```python
from build123d import *

# Parameters (mm, degrees)
CROQUIS1_R                 = 1.6
SALIENTE_EXTRUIR1_DEPTH    = 10
CORTAR_EXTRUIR1_DEPTH      = 8.1
CORTAR_EXTRUIR1_DEPTH_BACK = 8.1
CORTAR_EXTRUIR2_START      = 8.1
CROQUIS3_OUTSIDE_W         = 34.658
CROQUIS3_OUTSIDE_H         = 30.658
CROQUIS3_OUTSIDE_W_2       = 10
CROQUIS3_OUTSIDE_H_2       = 25.797501395
CORTAR_EXTRUIR2_DEPTH      = 8
CROQUIS4_W                 = 10
CROQUIS4_H                 = 8
SALIENTE_EXTRUIR3_DEPTH    = 3
CORTAR_EXTRUIR3_DEPTH      = 25.088378941
CORTAR_EXTRUIR3_DEPTH_BACK = 25.088378941
CROQUIS5_W                 = 8.1
CROQUIS5_H                 = 3.5
CROQUIS6_R                 = 4.5
CROQUIS6_R_2               = 1.6
SALIENTE_EXTRUIR4_DEPTH    = 3
CHAFL_N1_SIZE              = 1
CROQUIS7_R                 = 3.5
CORTAR_EXTRUIR4_DEPTH      = 3
SALIENTE_EXTRUIR8_START    = -1.9
CROQUIS8_R                 = 0.75
CROQUIS8_R_2               = 1.945
CROQUIS8_W                 = 23.65
CROQUIS8_H                 = 12.1
SALIENTE_EXTRUIR8_DEPTH    = 1.9
SALIENTE_EXTRUIR9_START    = 5
CROQUIS9_R                 = 1.945
SALIENTE_EXTRUIR9_DEPTH    = 5
CROQUIS10_W                = 23.280139212
CROQUIS10_H                = 3
SALIENTE_EXTRUIR10_DEPTH   = 11.4
CROQUIS11_R                = 1.945
SALIENTE_EXTRUIR11_DEPTH   = 2
REDONDEO1_R                = 3
CROQUIS12_W                = 4.35
CROQUIS12_H                = 6
CROQUIS12_R                = 0.75
SALIENTE_EXTRUIR12_DEPTH   = 2
CHAFL_N3_SIZE              = 2
CHAFL_N2_SIZE              = 1


# Some blends are built 0.0001 mm under size
with BuildPart() as part:
    # Croquis1 → Saliente-Extruir1 (new, symmetric)
    with BuildSketch(Plane.XY):
        with BuildLine():
            Line((-12.5, -15), (-5.566639674, 2.238866395))
            ThreePointArc((-5.566639674, 2.238866395), (0, 6), (5.566639674, 2.238866395))
            Line((5.566639674, 2.238866395), (12.5, -15))
            Line((12.5, -15), (-12.5, -15))
        make_face()
        Circle(CROQUIS1_R, mode=Mode.SUBTRACT)
    extrude(amount=SALIENTE_EXTRUIR1_DEPTH, both=True)

    # Croquis2 → Cortar-Extruir1 (cut, two sides: drawn at the far end of the back side and taken through both)
    with BuildSketch(Plane.XY.offset(-CORTAR_EXTRUIR1_DEPTH_BACK)):
        with BuildLine():
            Line((-12.5, -15), (-7.5, 0))
            ThreePointArc((-7.5, 0), (0, 7.5), (7.5, 0))
            Line((7.5, 0), (12.5, -15))
            Line((12.5, -15), (2.888582809, -8))
            Line((2.888582809, -8), (-3.164835235, -8))
            Line((-3.164835235, -8), (-12.5, -15))
        make_face()
    extrude(amount=CORTAR_EXTRUIR1_DEPTH + CORTAR_EXTRUIR1_DEPTH_BACK, mode=Mode.SUBTRACT)

    # Croquis3 outside → Cortar-Extruir2 (cut)
    with BuildSketch(Plane.XY.offset(CORTAR_EXTRUIR2_START)):
        with Locations((0, -4.5)):
            Rectangle(CROQUIS3_OUTSIDE_W, CROQUIS3_OUTSIDE_H)
        with Locations((0, -2.101249303)):
            Rectangle(CROQUIS3_OUTSIDE_W_2, CROQUIS3_OUTSIDE_H_2, mode=Mode.SUBTRACT)
    extrude(amount=-CORTAR_EXTRUIR2_DEPTH, mode=Mode.SUBTRACT)

    # Croquis4 → Saliente-Extruir3 (add)
    with BuildSketch(Plane.XZ.offset(15)):
        with Locations((0, 4.1)):
            Rectangle(CROQUIS4_W, CROQUIS4_H)
    extrude(amount=SALIENTE_EXTRUIR3_DEPTH)

    # Croquis5 → Cortar-Extruir3 (cut, two sides: drawn at the far end of the back side and taken through both)
    with BuildSketch(Plane(origin=(0, 0, 0), x_dir=(0, 0, -1), z_dir=(1, 0, 0)).offset(-CORTAR_EXTRUIR3_DEPTH_BACK)):
        with Locations((4.05, -9.75)):
            Rectangle(CROQUIS5_W, CROQUIS5_H)
    extrude(amount=CORTAR_EXTRUIR3_DEPTH + CORTAR_EXTRUIR3_DEPTH_BACK, mode=Mode.SUBTRACT)

    # Croquis6 → Saliente-Extruir4 (add)
    with BuildSketch(Plane.XY.offset(-8.1)):
        Circle(CROQUIS6_R)
        Circle(CROQUIS6_R_2, mode=Mode.SUBTRACT)
    extrude(amount=SALIENTE_EXTRUIR4_DEPTH)

    # Chaflán1
    chafl_n1_edges = [part.edges().sort_by_distance(p)[0] for p in [
        (-4.5, 0, -5.1),
    ]]
    chamfer(chafl_n1_edges, length=CHAFL_N1_SIZE)

    # Croquis7 → Cortar-Extruir4 (cut)
    with BuildSketch(Plane(origin=(0, 0, -10), x_dir=(-1, 0, 0), z_dir=(0, 0, -1))):
        Circle(CROQUIS7_R)
    extrude(amount=-CORTAR_EXTRUIR4_DEPTH, mode=Mode.SUBTRACT)

    # Croquis8 → Saliente-Extruir8 (add)
    with BuildSketch(Plane(origin=(0, 0, -10), x_dir=(-1, 0, 0), z_dir=(0, 0, -1)).offset(SALIENTE_EXTRUIR8_START)):
        with BuildLine():
            Line((65.2, -15), (65.2, 20.621697606))
            Line((65.2, 20.621697606), (30.587310575, 20.621717655))
            ThreePointArc((30.587310575, 20.621717655), (27.892014915, 20.154008561), (25.511873338, 18.805566286))
            Line((25.511873338, 18.805566286), (5.505516372, 2.38522315))
            ThreePointArc((5.505516372, 2.38522315), (5.536561655, 2.312246753), (5.566639674, 2.238866395))
            Line((5.566639674, 2.238866395), (12.5, -15))
            Line((12.5, -15), (65.2, -15))
        make_face()
        with Locations((59.747279072, 13.15)):
            Circle(CROQUIS8_R, mode=Mode.SUBTRACT)
        with Locations((31.747279072, 13.15)):
            Circle(CROQUIS8_R, mode=Mode.SUBTRACT)
        with Locations((22.280139212, 4.212923787)):
            Circle(CROQUIS8_R_2, mode=Mode.SUBTRACT)
        with Locations((45.747279072, 13.15)):
            Rectangle(CROQUIS8_W, CROQUIS8_H, mode=Mode.SUBTRACT)
    extrude(amount=SALIENTE_EXTRUIR8_DEPTH)

    # Croquis9 → Saliente-Extruir9 (add)
    with BuildSketch(Plane.XY.offset(-8.1).offset(SALIENTE_EXTRUIR9_START)):
        with BuildLine():
            Line((-27.280139212, -15), (-17.280139212, -15))
            Line((-17.280139212, -15), (-17.280139212, 10.371029295))
            ThreePointArc((-17.280139212, 10.371029295), (-22.280139212, 12.145279266), (-27.280139212, 10.371029295))
            Line((-27.280139212, 10.371029295), (-27.280139212, -15))
        make_face()
        with Locations(Location((-22.280139212, 4.212923787, 0), (0, 0, 180))):
            Circle(CROQUIS9_R, mode=Mode.SUBTRACT)
    extrude(amount=-SALIENTE_EXTRUIR9_DEPTH)

    # Croquis10 → Saliente-Extruir10 (add)
    with BuildSketch(Plane(origin=(0, 0, -10), x_dir=(-1, 0, 0), z_dir=(0, 0, -1))):
        with Locations((16.640069606, -13.5)):
            Rectangle(CROQUIS10_W, CROQUIS10_H)
    extrude(amount=SALIENTE_EXTRUIR10_DEPTH)

    # Croquis11 → Saliente-Extruir11 (add)
    with BuildSketch(Plane(origin=(0, 0, -21.4), x_dir=(-1, 0, 0), z_dir=(0, 0, -1))):
        Polygon((28.280139212, -15), (28.280139212, 10.566063957), (13.946510162, 10.566063957), (5, -12), (5, -15), align=None)
        with Locations((22.280139212, 4.212923787)):
            Circle(CROQUIS11_R, mode=Mode.SUBTRACT)
    extrude(amount=SALIENTE_EXTRUIR11_DEPTH)

    # Redondeo1
    redondeo1_edges = [part.edges().sort_by_distance(p)[0] for p in [
        (-65.2, 20.621697606, -9.05),
        (-28.280139212, 10.566063957, -22.4),
        (-13.946510162, 10.566063957, -22.4),
    ]]
    fillet(redondeo1_edges, radius=REDONDEO1_R)

    # Croquis12 → Saliente-Extruir12 (add)
    # profile 1 of 2: a face of its own
    with BuildSketch(Plane(origin=(0, 0, -10), x_dir=(-1, 0, 0), z_dir=(0, 0, -1))):
        with Locations((31.747279072, 13.15)):
            Rectangle(CROQUIS12_W, CROQUIS12_H)
        with Locations((31.747279072, 13.15)):
            Circle(CROQUIS12_R, mode=Mode.SUBTRACT)
    # profile 2 of 2: a face of its own
    with BuildSketch(Plane(origin=(0, 0, -10), x_dir=(-1, 0, 0), z_dir=(0, 0, -1))):
        with Locations((59.747279072, 13.15)):
            Rectangle(CROQUIS12_W, CROQUIS12_H)
        with Locations((59.747279072, 13.15)):
            Circle(CROQUIS12_R, mode=Mode.SUBTRACT)
    extrude(amount=SALIENTE_EXTRUIR12_DEPTH)

    # Chaflán3
    chafl_n3_edges = [part.edges().sort_by_distance(p)[0] for p in [
        (-31.747279072, 16.15, -10),
        (-31.747279072, 10.15, -10),
        (-59.747279072, 10.15, -10),
        (-59.747279072, 16.15, -10),
    ]]
    chamfer(chafl_n3_edges, length=CHAFL_N3_SIZE - 0.0001)  # a hair under: the kernel refuses the full size

    # Chaflán2
    # the kernel refuses this chamfer: 1 mm, written as the material it takes off along each edge
    with BuildSketch(Plane(origin=(0, 0, -10), x_dir=(-0.9997966291820871, -0.020166811253548467, 0), z_dir=(0.020166811253548467, -0.9997966291820871, 0))) as chafl_n2_piece_1_section:
        Polygon((6, -CHAFL_N2_SIZE), (6 - CHAFL_N2_SIZE, 0), (6, 0), align=None)
    chafl_n2_piece_1 = revolve(axis=Axis((0, 0, -10), (0, 0, -1)), revolution_arc=159.245879782, mode=Mode.PRIVATE)
    chafl_n2_piece_1 = split(chafl_n2_piece_1, bisect_by=Plane(origin=(-3.804583519, 0.989171828, -9.513770005), z_dir=(0.6344290754241263, 0.7729810788476574, 0)), keep=Keep.TOP, mode=Mode.PRIVATE)
    add(chafl_n2_piece_1, mode=Mode.SUBTRACT)
    with BuildSketch(Plane(origin=(5.566639674, 2.238866395, -10), x_dir=(0.02550993960358281, 0.01025993235875113, 0.9996219169112968), z_dir=(0.3731443992151493, -0.9277732790581789, 0))) as chafl_n2_piece_2:
        Polygon((CHAFL_N2_SIZE * 0.999621916911, CHAFL_N2_SIZE * 0.0274958766106), (-CHAFL_N2_SIZE * 0.0274958766106, CHAFL_N2_SIZE * 0.999621916911), (0, 0), align=None)
    extrude(amount=21.152587164, mode=Mode.SUBTRACT)


solid = part.part
```
Can you work these out from the model? Positions are in its coordinate system, mm. A direction names the side the tool comes from. Coordinates: 2 decimals unless noted, no trailing zeros. Write each loop counter-clockwise with the first axis right and the second up, starting at its lowest first coordinate (ties: lowest second). Pieces come first, ordered by that corner, then holes. Notation, with made-up numbers: (24, 26) - (28, 26) arc R23 cw to (28, 40) - close; hole circle Ø6 at (46.5, -0.5). An arc over 180 degrees is marked (long way). Return JSON: item names as keys, results as strings.
Q1. I'm going to push flat-ended pins straight in: pin 1 Ø5 at (x, y) = (-60.5, 13) entering from -Z; pin 2 Ø5 at (x, z) = (-3.5, -18) entering from -Y; pin 3 Ø6 at (y, z) = (-7.5, 3.5) entering from -X. Where does each tip first touch, or does it pass through?
Computed values:
{"pin 1": "stops at z = -12", "pin 2": "stops at y = -15", "pin 3": "stops at x = -5"}
Q2. On a 3-axis mill with a long thin cutter (end or side, diameter ignored), from which of +Z, -Z, +X, -X, +Y, -Y can I reach the whole of each face in a straight line? I mean faces 5 (the flat face through (0, -4, 8.1)), 6 (the flat face through (-7, -13, 0.1)), 7 (the flat face through (-16, -12, -16)). Say none if no direction works.
Computed values:
{"face 5": "+Y", "face 6": "-X, +Y, -Y", "face 7": "+X, -X, +Y"}
Q3. Please list where these lines run through material, in increasing order: L1, parallel to X at y = 13, z = -11; L2, parallel to Y at x = 0, z = -8; L3, parallel to Y at x = 0, z = -6.1. Write a range as from..to.
Computed values:
{"L1": "x = -61.92..-60.48, -59.01..-57.57, -33.92..-32.48, -31.01..-29.57", "L2": "y = -15..-11.5, -4.5..-3.5, 3.5..4.5", "L3": "y = -15..-11.5, -4.5..-1.6, 1.6..4.5"}
Q4. If we section it at D-D (z = 1): Please give me the cut outline in (x, y), then the cut area to 3 significant figures.
Computed values:
{"outline": "(-5, -18) - (5, -18) - (5, -9.54) - (2.89, -8) - (-3.16, -8) - (-5, -9.38) - close", "area": "97.1 mm2"}
Q5. If we section it at A-A (x = 0): Count the separate pieces of the cut face and the enclosed holes in it, then the cut area to 3 significant figures.
Computed values:
{"separate pieces": "3", "enclosed holes": "0", "area": "181 mm2"}
Q6. If we section it at C-C (y = 15): Please give me the cut outline in (x, z), then the cut area to 3 significant figures.
Computed values:
{"outline": "(-65.2, -10) - (-61.92, -10) - (-61.92, -12) - (-57.57, -12) - (-57.57, -8.1) - (-65.2, -8.1) - close; (-33.92, -12) - (-29.57, -12) - (-29.57, -10) - (-20.88, -10) - (-20.88, -8.1) - (-33.92, -8.1) - close", "area": "56.7 mm2"}
Q7. If we section it at B-B (x = -49): Please give me the cut outline in (y, z).
Computed values:
{"outline": "(-15, -10) - (7.1, -10) - (7.1, -8.1) - (-15, -8.1) - close; (19.2, -10) - (20.62, -10) - (20.62, -8.1) - (19.2, -8.1) - close"}
Q8. Thinking about a two-plate mould opening in Y: for faces 1 (the flat face through (-57.572, 13, -10)), 2 (the flat face through (8.83, -12.327, -1.913)), 3 (the flat face through (-33.922, 13, -10)), 4 (the flat face through (7, -13, 0.1)), which applies, +Y half, -Y half, draft (parallel to the pull), parting line (faces both ways), or undercut?
Computed values:
{"face 1": "undercut", "face 2": "+Y half", "face 3": "undercut", "face 4": "draft"}
